Input: part model. Units: mm. Frame: model coordinates. A direction names the side the tool comes from. Coordinates: 2 decimals unless noted, no trailing zeros. Order: outer loops, then holes, each group sorted by start corner. A loop starts at its lowest first (then second) coordinate and runs counter-clockwise, first axis right, second up.
from build123d import *

# Parameters (mm, degrees)
SKETCH_W        = 9.5
SKETCH_H        = 11.35
PAD_DEPTH       = 1.5
POCKET003_DEPTH = 0.5
FILLET006_R     = 0.25


with BuildPart() as part:
    # Sketch → Pad (new body)
    with BuildSketch(Plane.XY):
        with Locations((0, -0.825)):
            Rectangle(SKETCH_W, SKETCH_H)
    extrude(amount=PAD_DEPTH)

    # Sketch009 → Pocket003 (cut)
    with BuildSketch(Plane.XY):
        with BuildLine():
            Line((4.75, 4.85), (2.5, 4.85))
            Line((2.5, 4.85), (2.5, 3.425))
            ThreePointArc((2.5, 3.425), (2.792893, 2.717893), (3.5, 2.425))
            Line((3.5, 2.425), (4.75, 2.425))
            Line((4.75, 2.425), (4.75, 4.85))
        make_face()
        with BuildLine():
            Line((-3.5, -3.25), (-4.75, -3.25))
            Line((-4.75, -3.25), (-4.75, -5.25))
            Line((-3.5, -5.25), (-4.75, -5.25))
            ThreePointArc((-3.5, -5.25), (-2.792893, -4.957107), (-2.5, -4.25))
            ThreePointArc((-2.5, -4.25), (-2.792893, -3.542893), (-3.5, -3.25))
        make_face()
    extrude(amount=POCKET003_DEPTH, mode=Mode.SUBTRACT)

    # Fillet006
    fillet006_edges = [part.edges().sort_by_distance(p)[0] for p in [
        (4.75, 4.85, 1),
        (4.75, -6.5, 0.75),
        (-4.75, -6.5, 0.75),
        (-4.75, 4.85, 0.75),
    ]]
    fillet(fillet006_edges, radius=FILLET006_R)


solid = part.part
Item 1: Ray query, probe 1 along Z at (x, y) = (4.25, 4); probe 2 along X at (y, z) = (3, 0.25); probe 3 along X at (y, z) = (4.75, 0.35). Return the intervals inside material, ascending.
Response values:
probe 1: z = 0.5 to 1.5
probe 2: x = -4.75 to 2.59
probe 3: x = -4.7 to 2.5
Item 2: Draft query along Y for faces 3 (the face through (0, 4.85, 1)), 4 (the face through (0, -1, 1.5)), 5 (the face through (0, -6.5, 1)), 6 (the face through (-4, -4, 0.5)). Return one class per face: pulls with the +Y half, pulls with the -Y half, needs draft (parallel to the pull), parting line crosses it, or undercut.
Response values:
face 3: pulls with the +Y half
face 4: needs draft
face 5: pulls with the -Y half
face 6: undercut
Item 3: Cut plane B-B on x = 4.25. Return loops of the section in (y, z) (3 decimals), then the cut area to 3 significant figures.
Response values:
outline: (-6.5, 0) - (2.425, 0) - (2.425, 0.5) - (4.85, 0.5) - (4.85, 1.5) - (-6.5, 1.5) - close
area: 15.8 mm2
Item 4: Cut plane A-A on y = 4. Return loops of the section in (x, z).
Response values:
outline: (-4.75, 0) - (2.5, 0) - (2.5, 0.5) - (4.75, 0.5) - (4.75, 1.5) - (-4.75, 1.5) - close
Item 5: Pin query (flat end, axial travel): pin 1 Ø1.6 at (x, y) = (-4, -4.5) entering from -Z; pin 2 Ø0.7 at (x, y) = (3.5, 4) entering from -Z. Return the tip coordinate at first contact, or that it passes through.
Response values:
pin 1: stops at z = 0
pin 2: stops at z = 0.5
Item 6: Access query for faces 1 (the face through (4.75, -1, 1)), 2 (the face through (4, 4, 0.5)). Directions: +Z, -Z, +X, -X, +Y, -Y. A direction counts if a zero-diameter tool reaches every point of the face in a straight line with its end or side. Return the directions, or none.
Response values:
face 1: +Z, -Z, +X, +Y, -Y
face 2: -Z, +X, +Y
